from build123d import *

# Parameters (mm, degrees)
F0_W     = 152
F0_H     = 120
F1_DEPTH = 27
F3_DEPTH = 120.001


with BuildPart() as f1:
    # F0 (on Top) → F1 (new body)
    with BuildSketch(Plane.XY):
        Rectangle(F0_W, F0_H)
    extrude(amount=F1_DEPTH)

    # F2 (on face) → F3 (cut, through all)
    with BuildSketch(Plane(origin=(0, 60, 0), x_dir=(-1, 0, 0), z_dir=(0, 1, 0))):
        Polygon((-76, 20.25), (-68, 27), (-76, 27), align=None)
        Polygon((-76, 0), (-68, 0), (-76, 6.75), align=None)
        Polygon((76, 6.75), (68, 0), (76, 0), align=None)
        Polygon((76, 27), (68, 27), (76, 20.25), align=None)
    extrude(amount=-F3_DEPTH, mode=Mode.SUBTRACT)


solid = f1.part
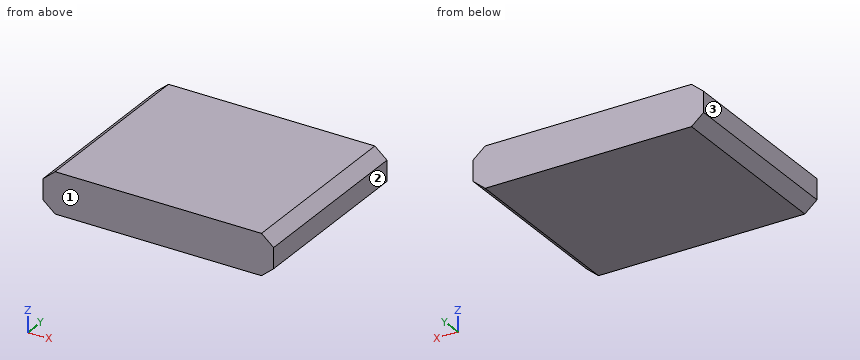
Part model, mm, in its own coordinate system. Face numbers are marked on the shaded views. Coordinates: 2 decimals unless noted, no trailing zeros. Order: outer loops, then holes, each group sorted by start corner. A loop starts at its lowest first (then second) coordinate and runs counter-clockwise, first axis right, second up.
(1) Pull direction X, two halves, no side cores. Call the marked faces 1, 2 and 3: pulls with the +X half, pulls with the -X half, needs draft (parallel to the pull), parting line crosses it, or undercut.
Check sheet entries:
face 1: needs draft
face 2: pulls with the +X half
face 3: pulls with the -X half
(2) Pin check, flat tip, straight feed: pin 1 Ø1.5 at (x, y) = (44.5, 43) entering from -Z. Stop position of the tip, or through.
Check sheet entries:
pin 1: stops at z = 0
(3) Slice it at B-B, the plane z = 24. Write the cut outline in (x, y).
Check sheet entries:
outline: (-71.56, -60) - (71.56, -60) - (71.56, 60) - (-71.56, 60) - close
(4) Slice it at A-A, the plane y = -24. Write the cut outline in (x, z).
Check sheet entries:
outline: (-76, 6.75) - (-68, 0) - (68, 0) - (76, 6.75) - (76, 20.25) - (68, 27) - (-68, 27) - (-76, 20.25) - close
(5) Slice it at C-C, the plane z = 5. Write the cut outline in (x, y), and give its area (3 significant figures).
Check sheet entries:
outline: (-73.93, -60) - (73.93, -60) - (73.93, 60) - (-73.93, 60) - close
area: 17,700 mm2
(6) Probe L1, parallel to X at y = -3, z = 22; L2, parallel to X at y = 0, z = 23.75. List the from-to ranges inside material, lowest first.
Check sheet entries:
L1: x = -73.93 to 73.93
L2: x = -71.85 to 71.85
